from build123d import *

# Parameters (mm, degrees)
SKETCH1_W           = 43
SKETCH1_H           = 25.6
SKETCH1_R           = 3.2305
BOSS_EXTRUDE1_DEPTH = 7
BOSS_EXTRUDE2_DEPTH = 6
FILLET1_R           = 6
BOSS_EXTRUDE3_REACH = 57.854
SKETCH3_W           = 16
SKETCH3_H           = 25.6
FILLET2_R           = 3
FILLET3_R           = 2


with BuildPart() as part:
    # Sketch1 → Boss-Extrude1 (new body)
    with BuildSketch(Plane(origin=(0, 0, 0), x_dir=(1, 0, 0), z_dir=(0, 1, 0))):
        Rectangle(SKETCH1_W, SKETCH1_H)
        with Locations(Location((-8.8, 0, 0), (0, 0, 270))):
            Circle(SKETCH1_R, mode=Mode.SUBTRACT)
        with Locations(Location((11.2, 0, 0), (0, 0, 270))):
            Circle(SKETCH1_R, mode=Mode.SUBTRACT)
    extrude(amount=BOSS_EXTRUDE1_DEPTH)

    # Sketch2 → Boss-Extrude2 (add)
    with BuildSketch(Plane.XY.offset(12.8)):
        Polygon((21.5, 7), (21.5, 0), (-21.5, 0), (-21.5, 7), (-21.5, 55), (-1.5, 55), align=None)
        with BuildLine():
            Line((-10.8, 50.5), (-6.8, 50.5))
            ThreePointArc((-6.8, 50.5), (-3.3, 47), (-6.8, 43.5))
            Line((-6.8, 43.5), (-10.8, 43.5))
            ThreePointArc((-10.8, 43.5), (-14.3, 47), (-10.8, 50.5))
        make_face(mode=Mode.SUBTRACT)
        with BuildLine():
            Line((-10.8, 22.5), (-6.8, 22.5))
            ThreePointArc((-6.8, 22.5), (-3.3, 19), (-6.8, 15.5))
            Line((-6.8, 15.5), (-10.8, 15.5))
            ThreePointArc((-10.8, 15.5), (-14.3, 19), (-10.8, 22.5))
        make_face(mode=Mode.SUBTRACT)
    boss_extrude2 = extrude(amount=BOSS_EXTRUDE2_DEPTH)

    # Mirror1: Boss-Extrude2 across plane
    add(boss_extrude2.mirror(Plane.XY))

    # Fillet1
    fillet1_edges = [part.edges().sort_by_distance(p)[0] for p in [
        (-1.5, 55, 15.8),
        (-21.5, 55, 15.8),
        (-1.5, 55, -15.8),
        (-21.5, 55, -15.8),
    ]]
    fillet(fillet1_edges, radius=FILLET1_R)

    # Boss-Extrude3: up to this face of the body (flat: up to its plane)
    boss_extrude3_end = Plane(part.part.faces().sort_by_distance((10.816327241, 29.296360541, -15.8))[0])
    # Sketch3 → Boss-Extrude3 (add, up to the picked face)
    with BuildSketch(Plane(origin=(0, 7, 0), x_dir=(1, 0, 0), z_dir=(0, 1, 0)), mode=Mode.PRIVATE) as boss_extrude3_sk1:
        with Locations((13.5, 0)):
            Rectangle(SKETCH3_W, SKETCH3_H)
    boss_extrude3_tool1 = split(extrude(boss_extrude3_sk1.sketch, amount=BOSS_EXTRUDE3_REACH, mode=Mode.PRIVATE), bisect_by=boss_extrude3_end, keep=Keep.BOTH, mode=Mode.PRIVATE)
    add(boss_extrude3_tool1.solids().sort_by(Axis((13.5, 7, 0), (0, 1, 0)))[0])

    # Fillet2
    fillet2_edges = [part.edges().sort_by_distance(p)[0] for p in [
        (5.5, 40.391304348, 0),
    ]]
    fillet(fillet2_edges, radius=FILLET2_R)

    # Fillet3
    fillet3_edges = [part.edges().sort_by_distance(p)[0] for p in [
        (-2.081080958, 54.077220031, 18.8),
        (-19.742640687, 53.242640687, 18.8),
        (5.669051284, 40.038501669, -12.8),
        (5.669051284, 40.038501669, 12.8),
        (10.816327241, 29.296360541, 18.8),
        (21.5, 3.5, 18.8),
        (21.5, 7, 0),
        (10.816327241, 29.296360541, -18.8),
        (21.5, 3.5, -18.8),
        (-10.389120846, 55, -12.8),
        (-10.389120846, 55, -18.8),
        (-21.5, 28, -12.8),
        (-2.081080958, 54.077220031, -12.8),
        (-19.742640687, 53.242640687, -12.8),
        (-21.5, 24.5, 18.8),
        (-21.5, 28, 12.8),
        (-21.5, 24.5, -18.8),
        (-2.081080958, 54.077220031, -18.8),
        (-19.742640687, 53.242640687, -18.8),
        (-10.389120846, 55, 12.8),
        (-2.081080958, 54.077220031, 12.8),
        (-19.742640687, 53.242640687, 12.8),
        (-10.389120846, 55, 18.8),
    ]]
    fillet(fillet3_edges, radius=FILLET3_R)


solid = part.part
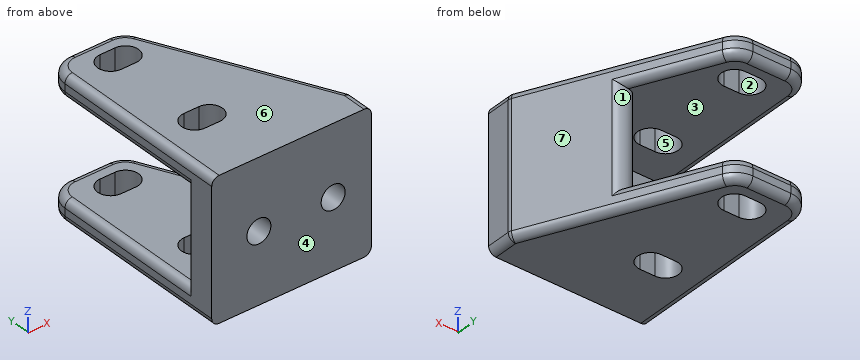
Part model, mm, in its own coordinate system. Face numbers are marked on the shaded views. A direction names the side the tool comes from. Coordinates: 2 decimals unless noted, no trailing zeros. Order: outer loops, then holes, each group sorted by start corner. A loop starts at its lowest first (then second) coordinate and runs counter-clockwise, first axis right, second up. Notation, with made-up numbers: M -16.5,33.5 L 27.5,33.5 A33 cw 27.5,71.5 Z; hole C 42.25,22.25 d4. An arc over 180 degrees is marked long. One line per question, with ' | ' between items.
Q1. Slice it at B-B (z = 4.5). Give the cut face in (x, y), and give its area (3 significant figures).
A:
outline: M -21.5,0 L 21.5,0 L 21.5,6.55 A2 ccw 21.3,7.41 L 11.21,28.48 A3 ccw 5.5,27.19 L 5.5,7 L -21.5,7 Z | area: 541 mm^2
Q2. Slice it at A-A (x = -8.8). Count the separate pieces of the cut face and the enclosed holes in it, and give its area (3 significant figures).
A:
separate pieces: 6 | enclosed holes: 0 | area: 623 mm^2
Q3. Drill centre lines: line 1 (X direction, y = 2.75, z = 0); line 2 (Z direction, x = -8, y = 23.5); line 3 (Z direction, x = 11, y = 3). Where is each one in solid material? Low to high.
A:
line 1: x = -21.5 to -12.03, -5.57 to 7.97, 14.43 to 21.5 | line 2: z = -18.8 to -12.8, 12.8 to 18.8 | line 3: z = -18.8 to -3.22, 3.22 to 18.8
Q4. Pin check, flat tips, straight feed: P1, Ø1, axis at y = 28, z = -2.5, coming from the +X side; P2, Ø4, axis at x = -8.8, z = 0, coming from the +Y side; P3, Ø8, axis at x = 12, z = -8.5, coming from the +Y side; P4, Ø1.9, axis at x = 10.5, z = -1.5, coming from the -Y side. Stop position of each tip, or through.
A:
P1: stops at x = 11.68 | P2: passes through | P3: stops at y = 30.19 | P4: stops at y = 7
Q5. Slice it at C-C (z = 0). Give the cut face in (x, y).
A:
outline: M -21.5,0 L -12.03,0 L -12.03,7 L -21.5,7 Z; M -5.57,0 L 7.97,0 L 7.97,7 L 14.43,7 L 14.43,0 L 21.5,0 L 21.5,6.55 A2 ccw 21.3,7.41 L 11.21,28.48 A3 ccw 5.5,27.19 L 5.5,7 L -5.57,7 Z
Q6. Two-plate mould, pull along Y, no slides. Class the marked faces 4, 5, 6 and 7: +Y half, -Y half, draft (parallel to the pull), parting line (faces both ways), or undercut.
A:
face 4: -Y half | face 5: undercut | face 6: draft | face 7: +Y half
Q7. 3-axis set-ups, long thin cutter, end or side, ignore diameter. For the marked faces 1, 2 and 3: which of +Z, -Z, +X, -X, +Y, -Y reach the whole face in a straight line?
A:
face 1: +Y | face 2: +Z, -Z | face 3: -X, +Y
